Read the model definition and answer for the solid it produces. Units are mm, in the model's axes. Face numbers are marked on the shaded views. A direction names the side the tool comes from. Give positions to 0.01 mm unless a question says otherwise; leave off trailing zeros. Loops run counter-clockwise (first coordinate to the right, second up) from the corner with the lowest first, then second, coordinate; pieces in that order, holes last. Notation, with made-up numbers: (58.5, -4) - (83.5, -4) arc R26 ccw to (83.5, 35) - close; hole circle Ø11 at (-10.75, -5). An arc over 180 degrees is marked (long way). Use a Markdown table: item, result. Add a question column.
Item 1: Consider probe 1 along Y at (x, z) = (10.5, 8.25); probe 2 along Y at (x, z) = (0.75, -7); probe 3 along Z at (x, y) = (-9.5, 0.5). Determine where each line is inside the solid, lowest interval first. Write a range as [from, to].
Item 2: For a pull along X with two mould halves and no side action, classify the marked faces 1, 2 and 3 as +X half, -X half, draft (parallel to the pull), parting line (faces both ways), or undercut.
Item 3: A cutting plane is placed at A-A (y = -2). Determine the outline of the cut face in (x, z).
Item 4: Each of these flat-tipped pins is pushed along its axis until it touches: P1, Ø6, axis at y = 9, z = -9, coming from the -X side; P2, Ø1, axis at x = -8.5, z = -10, coming from the -Y side; P3, Ø6, axis at x = -8.5, y = 10.5, coming from the -Z side; P4, Ø1.5, axis at y = 29, z = -4, coming from the +X side. Where does it stop, or does it pass through?
Item 5: A cutting plane is placed at C-C (x = 7). Determine the outline of the cut face in (y, z).
Item 6: A cutting plane is placed at B-B (z = 0). Determine the outline of the cut face in (x, y).
Item 7: Which of the six approach directions +Z, -Z, +X, -X, +Y, -Y give full straight-line access (tool end or side, diameter ignored) to the marked faces 4, 5 and 6?
Item 8: A cutting plane is placed at D-D (y = 29). Determine the outline of the cut face in (x, z).
from build123d import *

# Parameters (mm, degrees)
ESQUISSE1_R        = 14
BOSS_EXTRU_1_DEPTH = 20
ESQUISSE2_R        = 2.5
BOSS_EXTRU_2_DEPTH = 15
ESQUISSE3_R        = 1.5
ESQUISSE3_R_2      = 1.438113866
BOSS_EXTRU_3_DEPTH = 5


with BuildPart() as part:
    # Esquisse1 → Boss.-Extru.1 (new body)
    with BuildSketch(Plane(origin=(0, 0, 0), x_dir=(1, 0, 0), z_dir=(0, 1, 0))):
        with Locations(Location((0, 0, 0), (0, 0, 270))):
            Circle(ESQUISSE1_R)
    extrude(amount=BOSS_EXTRU_1_DEPTH)

    # Esquisse2 → Boss.-Extru.2 (add)
    with BuildSketch(Plane(origin=(0, 20, 0), x_dir=(1, 0, 0), z_dir=(0, 1, 0))):
        with Locations(Location((0, 0, 0), (0, 0, 270))):
            Circle(ESQUISSE2_R)
    extrude(amount=BOSS_EXTRU_2_DEPTH)

    # Esquisse3 → Boss.-Extru.3 (add)
    with BuildSketch(Plane(origin=(0, 0, 0), x_dir=(-1, 0, 0), z_dir=(0, -1, 0))):
        with Locations(Location((-8, 0, 0), (0, 0, 270))):
            Circle(ESQUISSE3_R)
        with Locations(Location((0, 8, 0), (0, 0, 270))):
            Circle(ESQUISSE3_R)
        with Locations(Location((8, 0, 0), (0, 0, 270))):
            Circle(ESQUISSE3_R_2)
        with Locations(Location((0, -8, 0), (0, 0, 270))):
            Circle(ESQUISSE3_R)
    extrude(amount=BOSS_EXTRU_3_DEPTH)


solid = part.part
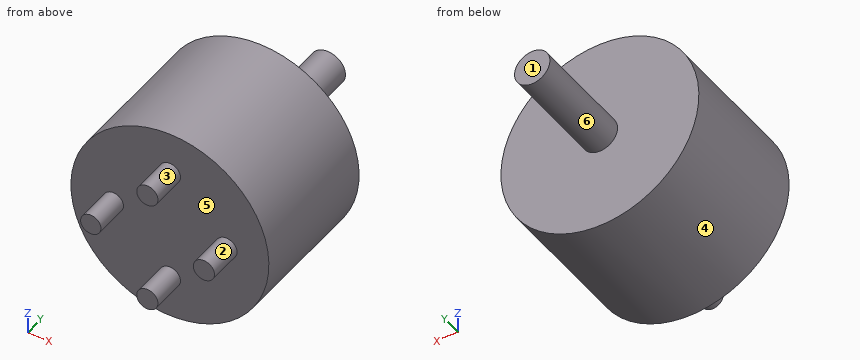
Geometry says:
| question | item | result |
|---|---|---|
| 1 | probe 1 | [0, 20] |
| 1 | probe 2 | [-5, 20] |
| 1 | probe 3 | [-10.28, 10.28] |
| 2 | face 1 | draft |
| 2 | face 2 | undercut |
| 2 | face 3 | parting line |
| 3 | outline | circle Ø2.88 at (-8, 0); circle Ø3 at (0, -8); circle Ø3 at (0, 8); circle Ø3 at (8, 0) |
| 4 | P1 | x = -12.65 |
| 4 | P2 | y = 0 |
| 4 | P3 | z = -12.87 |
| 4 | P4 | through |
| 5 | outline | (-5, -1.12) - (0, -1.12) - (0, -12.12) - (20, -12.12) - (20, 12.12) - (0, 12.12) - (0, 1.12) - (-5, 1.12) - close |
| 6 | outline | (-14, 0) - (-9.44, 0) - (-9.44, -5) - (-6.56, -5) - (-6.56, 0) - (6.5, 0) - (6.5, -5) - (9.5, -5) - (9.5, 0) - (14, 0) - (14, 20) - (2.5, 20) - (2.5, 35) - (-2.5, 35) - (-2.5, 20) - (-14, 20) - close |
| 7 | face 4 | +Y, -Y |
| 7 | face 5 | -Y |
| 7 | face 6 | +Y |
| 8 | outline | circle Ø5 at (0, 0) |
